Build history of the part. All positions in model axes, mm. Round coordinates to 2 decimals unless told otherwise and drop trailing zeros. Order: outer loops, then holes, each group sorted by start corner. A loop starts at its lowest first (then second) coordinate and runs counter-clockwise, first axis right, second up. Notation, with made-up numbers: M -19.5,60 L 28.5,60 A29 ccw 28.5,86 Z; hole C 6,-12.5 d10. An arc over 180 degrees is marked long. One line per item, written item: value. Start each with the question number.
Item 1: Pin check, flat tips, straight feed: pin 1 (0.6 mm diameter, centred on y = 85.5, z = 1, fed in from +X); pin 2 (4 mm diameter, centred on x = 42.05, y = -2.52, fed in from +Z); pin 3 (0.9 mm diameter, centred on x = 2.5, z = 1.5, fed in from -Y); pin 4 (1.6 mm diameter, centred on x = -3.5, z = 1, fed in from +Y). Stop position of each tip, or through.
Item 2: Probe L1, parallel to Y at x = 98.25, z = 1.3; L2, parallel to X at y = -59, z = 2.9; L3, parallel to Y at x = 42.5, z = 2.85. List the from-to ranges inside material, lowest first.
Item 3: Two-plate mould, pull along Y, no slides. Class faces 1 (the flat face through (-1, 1, 0)), 2 (the cylindrical face through (-13.713, -1.469, 1.612)): +Y half, -Y half, draft (parallel to the pull), parting line (faces both ways), or undercut.
Item 4: Band-saw the part on A-A, the plane y = -39. Write the cut outline in (x, z), then the cut area to 3 significant figures.
Item 5: Band-saw the part on B-B, the plane z = 2.35. Give the number of separate pieces and of enclosed holes in the cut face, then the cut area to 3 significant figures.
```python
from build123d import *

# Parameters (mm, degrees)
SKETCH2_W           = 193.64
SKETCH2_H           = 180
BOSS_EXTRUDE1_DEPTH = 3.18
CUT_EXTRUDE1_DEPTH  = 133.227927459
SKETCH4_W           = 3.18
SKETCH4_H           = 10
BOSS_EXTRUDE2_DEPTH = 3.18
SKETCH6_R           = 1.47
CUT_EXTRUDE2_DEPTH  = 135.573817662
SKETCH7_R           = 3.5
CUT_EXTRUDE3_DEPTH  = 135.573817662
SKETCH9_W           = 2.024123771
SKETCH9_H           = 3.5
SKETCH9_W_2         = 2.024123772
CUT_EXTRUDE4_DEPTH  = 135.573817662


with BuildPart() as part:
    # Sketch2 → Boss-Extrude1 (new body)
    with BuildSketch(Plane.XY):
        Rectangle(SKETCH2_W, SKETCH2_H)
    extrude(amount=BOSS_EXTRUDE1_DEPTH)

    # Sketch3 → Cut-Extrude1 (cut, through all)
    with BuildSketch(Plane.XY.offset(3.18)):
        Polygon((-5, 90), (5, 90), (5, 86.82), (1.47, 86.82), (1.47, 84.74), (3.25, 84.74), (3.25, 82.14), (1.47, 82.14), (1.47, 80.07), (-1.47, 80.07), (-1.47, 82.14), (-3.25, 82.14), (-3.25, 84.74), (-1.47, 84.74), (-1.47, 86.82), (-5, 86.82), align=None)
        Polygon((1.47, -86.82), (5, -86.82), (5, -90), (-5, -90), (-5, -86.82), (-1.47, -86.82), (-1.47, -84.74), (-3.25, -84.74), (-3.25, -82.14), (-1.47, -82.14), (-1.47, -80.07), (1.47, -80.07), (1.47, -82.14), (3.25, -82.14), (3.25, -84.74), (1.47, -84.74), align=None)
    extrude(amount=-CUT_EXTRUDE1_DEPTH, mode=Mode.SUBTRACT)

    # Sketch4 → Boss-Extrude2 (add)
    with BuildSketch(Plane.ZY.offset(96.82)):
        with Locations((1.59, 0)):
            Rectangle(SKETCH4_W, SKETCH4_H)
    boss_extrude2 = extrude(amount=BOSS_EXTRUDE2_DEPTH)

    # Sketch6 → Cut-Extrude2 (cut, through all)
    with BuildSketch(Plane.XY.offset(3.18)):
        with Locations((-98.25, 0)):
            Circle(SKETCH6_R)
    cut_extrude2 = extrude(amount=-CUT_EXTRUDE2_DEPTH, mode=Mode.SUBTRACT)

    # Mirror1: Boss-Extrude2 across plane
    add(boss_extrude2.mirror(Plane(origin=(0, 0, 0), x_dir=(0, 0, 1), z_dir=(1, 0, 0))))

    # Mirror2: Cut-Extrude2 across plane
    add(cut_extrude2.mirror(Plane(origin=(0, 0, 0), x_dir=(0, 0, 1), z_dir=(1, 0, 0))), mode=Mode.SUBTRACT)

    # Sketch7 → Cut-Extrude3 (cut, through all)
    with BuildSketch(Plane.XY.offset(3.18)):
        with Locations((-51.119653384, -2.520413941)):
            Circle(SKETCH7_R)
        with Locations((-17.051323135, -2.520413941)):
            Circle(SKETCH7_R)
        with Locations((42.052504626, -2.520413941)):
            Circle(SKETCH7_R)
        with Locations((76.120834875, -2.520413941)):
            Circle(SKETCH7_R)
    extrude(amount=-CUT_EXTRUDE3_DEPTH, mode=Mode.SUBTRACT)

    # Sketch9 → Cut-Extrude4 (cut, through all)
    with BuildSketch(Plane(origin=(0, 0, 0), x_dir=(-1, 0, 0), z_dir=(0, 0, -1))):
        with Locations((59.039301131, -2.520413941)):
            Rectangle(SKETCH9_W, SKETCH9_H)
        with Locations((24.970970881, -2.520413941)):
            Rectangle(SKETCH9_W_2, SKETCH9_H)
        with Locations((-34.13285688, -2.520413941)):
            Rectangle(SKETCH9_W_2, SKETCH9_H)
        with Locations((-68.201187129, -2.520413941)):
            Rectangle(SKETCH9_W_2, SKETCH9_H)
    extrude(amount=-CUT_EXTRUDE4_DEPTH, mode=Mode.SUBTRACT)


solid = part.part
```
Output:
1. pin 1: stops at x = 96.82
1. pin 2: passes through
1. pin 3: stops at y = -86.82
1. pin 4: stops at y = 86.82
2. L1: y = -5 to -1.47, 1.47 to 5
2. L2: x = -96.82 to 96.82
2. L3: y = -90 to -5.99, 0.95 to 90
3. face 1: draft
3. face 2: undercut
4. outline: M -96.82,0 L 96.82,0 L 96.82,3.18 L -96.82,3.18 Z
4. area: 616 mm²
5. separate pieces: 1
5. enclosed holes: 10
5. area: 34,600 mm²
